Can you work these out from the model? Positions are in its coordinate system, mm. Face numbers are marked on the shaded views. A direction names the side the tool comes from. Give positions to 0.01 mm unless a question says otherwise; leave off trailing zeros. Return JSON: item names as keys, results as strings.
```python
from build123d import *

# Parameters (mm, degrees)
OUTER_R                               = 19.05
BODY_DEPTH                            = 4.7625
F_4_40_TAPPED_HOLE_D                  = 2.2606
SCREW_HOLES_COUNT                     = 4
F_43_0_089_DIAMETER_HOLE1_D           = 2.2606
F_1_8_0_125_DIAMETER_HOLE1_AT_2_COUNT = 2
F_1_8_0_125_DIAMETER_HOLE1_AT_2_PITCH = 19.763158772
F_1_8_0_125_DIAMETER_HOLE2_AT_2_COUNT = 2
F_1_8_0_125_DIAMETER_HOLE2_AT_2_PITCH = 19.763158772
IO_HOLES_PATTERN_COUNT                = 4
INSET_R                               = 19.05
INSET_R_2                             = 11.938
INSET_CUT_DEPTH                       = 1.016
POST_BOTTOMS_COUNT                    = 4
FLAT_CUT_SKETCH_W                     = 2.54
FLAT_CUT_SKETCH_H                     = 38.1
FLAT_CUT_DEPTH                        = 28.358479604


# Read off the part's stored shape, not the designer's step: #36 (0.1065) Diameter Hole1
with BuildPart() as part:
    # outer → Body (new body)
    with BuildSketch(Plane(origin=(0, 0, 0), x_dir=(1, 0, 0), z_dir=(0, 1, 0))):
        with Locations(Location((0, 0, 0), (0, 0, 270))):
            Circle(OUTER_R)
    extrude(amount=-BODY_DEPTH)

    # #4-40 Tapped Hole (through all)
    with Locations(Plane(origin=(0, 0, 0), x_dir=(1, 0, 0), z_dir=(0, 1, 0))):
        with Locations((-11.85393808, 11.85393808)):
            f_4_40_tapped_hole = Hole(F_4_40_TAPPED_HOLE_D / 2)

    # Screw Holes: #4-40 Tapped Hole ×4 about axis
    screw_holes_axis = Axis((0, 0, 0), (0, 1, 0))
    for i in range(1, SCREW_HOLES_COUNT):
        add(f_4_40_tapped_hole.rotate(screw_holes_axis, i * 360 / SCREW_HOLES_COUNT), mode=Mode.SUBTRACT)

    # #43 (0.089) Diameter Hole1 (through all)
    with Locations(Plane(origin=(0, 0, 0), x_dir=(1, 0, 0), z_dir=(0, 1, 0))):
        with Locations((-2.3622, 9.881579386), (-2.3622, -9.881579386)):
            f_43_0_089_diameter_hole1 = Hole(F_43_0_089_DIAMETER_HOLE1_D / 2)

    # Sketch40 → 1/8 (0.125) Diameter Hole1 (revolve, cut)
    with BuildSketch(Plane(origin=(-2.3622, 0, -9.881579386), x_dir=(0, 0, 1), z_dir=(1, 0, 0))):
        Polygon((0, 0), (0, 2.477866233), (1.5875, 1.524), (1.5875, 0), align=None)
    f_1_8_0_125_diameter_hole1 = revolve(axis=Axis((-2.3622, 6.35, -9.881579386), (0, -1, 0)), mode=Mode.SUBTRACT)

    # 1/8 (0.125) Diameter Hole1 at 2: 1/8 (0.125) Diameter Hole1 ×2
    with Locations(*[(0, 0, i * F_1_8_0_125_DIAMETER_HOLE1_AT_2_PITCH) for i in range(1, F_1_8_0_125_DIAMETER_HOLE1_AT_2_COUNT)]):
        add(f_1_8_0_125_diameter_hole1, mode=Mode.SUBTRACT)

    # Sketch42 → 1/8 (0.125) Diameter Hole2 (revolve, cut)
    with BuildSketch(Plane(origin=(-2.3622, -4.7625, -9.881579386), x_dir=(0, 0, -1), z_dir=(1, 0, 0))):
        Polygon((0, 0), (0, 2.477866233), (1.5875, 1.524), (1.5875, 0), align=None)
    f_1_8_0_125_diameter_hole2 = revolve(axis=Axis((-2.3622, -11.1125, -9.881579386), (0, 1, 0)), mode=Mode.SUBTRACT)

    # 1/8 (0.125) Diameter Hole2 at 2: 1/8 (0.125) Diameter Hole2 ×2
    with Locations(*[(0, 0, i * F_1_8_0_125_DIAMETER_HOLE2_AT_2_PITCH) for i in range(1, F_1_8_0_125_DIAMETER_HOLE2_AT_2_COUNT)]):
        add(f_1_8_0_125_diameter_hole2, mode=Mode.SUBTRACT)

    # IO Holes Pattern: #43 (0.089) Diameter Hole1, 1/8 (0.125) Diameter Hole1, 1/8 (0.125) Diameter Hole2 ×4 about axis
    io_holes_pattern_axis = Axis((0, 0, 0), (0, 1, 0))
    add([f_43_0_089_diameter_hole1.rotate(io_holes_pattern_axis, i * 360 / IO_HOLES_PATTERN_COUNT) for i in range(1, IO_HOLES_PATTERN_COUNT)], mode=Mode.SUBTRACT)
    add([f_1_8_0_125_diameter_hole1.rotate(io_holes_pattern_axis, i * 360 / IO_HOLES_PATTERN_COUNT) for i in range(1, IO_HOLES_PATTERN_COUNT)], mode=Mode.SUBTRACT)
    add([f_1_8_0_125_diameter_hole2.rotate(io_holes_pattern_axis, i * 360 / IO_HOLES_PATTERN_COUNT) for i in range(1, IO_HOLES_PATTERN_COUNT)], mode=Mode.SUBTRACT)

    # IO Holes Pattern copy 1 sketch → IO Holes Pattern copy 1 (revolve, cut)
    with BuildSketch(Plane(origin=(9.881579386, 0, 2.3622), x_dir=(1, 0, 0), z_dir=(0, 0, -1))):
        Polygon((0, 0), (0, 2.477866233), (1.5875, 1.524), (1.5875, 0), align=None)
    revolve(axis=Axis((9.881579386, 6.35, 2.3622), (0, -1, 0)), mode=Mode.SUBTRACT)

    # IO Holes Pattern copy 2 sketch → IO Holes Pattern copy 2 (revolve, cut)
    with BuildSketch(Plane(origin=(2.3622, 0, -9.881579386), x_dir=(0, 0, -1), z_dir=(-1, 0, 0))):
        Polygon((0, 0), (0, 2.477866233), (1.5875, 1.524), (1.5875, 0), align=None)
    revolve(axis=Axis((2.3622, 6.35, -9.881579386), (0, -1, 0)), mode=Mode.SUBTRACT)

    # IO Holes Pattern copy 3 sketch → IO Holes Pattern copy 3 (revolve, cut)
    with BuildSketch(Plane(origin=(-9.881579386, 0, -2.3622), x_dir=(-1, 0, 0), z_dir=(0, 0, 1))):
        Polygon((0, 0), (0, 2.477866233), (1.5875, 1.524), (1.5875, 0), align=None)
    revolve(axis=Axis((-9.881579386, 6.35, -2.3622), (0, -1, 0)), mode=Mode.SUBTRACT)

    # IO Holes Pattern copy 4 sketch → IO Holes Pattern copy 4 (revolve, cut)
    with BuildSketch(Plane(origin=(9.881579386, -4.7625, 2.3622), x_dir=(-1, 0, 0), z_dir=(0, 0, -1))):
        Polygon((0, 0), (0, 2.477866233), (1.5875, 1.524), (1.5875, 0), align=None)
    revolve(axis=Axis((9.881579386, -11.1125, 2.3622), (0, 1, 0)), mode=Mode.SUBTRACT)

    # IO Holes Pattern copy 5 sketch → IO Holes Pattern copy 5 (revolve, cut)
    with BuildSketch(Plane(origin=(2.3622, -4.7625, -9.881579386), x_dir=(0, 0, 1), z_dir=(-1, 0, 0))):
        Polygon((0, 0), (0, 2.477866233), (1.5875, 1.524), (1.5875, 0), align=None)
    revolve(axis=Axis((2.3622, -11.1125, -9.881579386), (0, 1, 0)), mode=Mode.SUBTRACT)

    # IO Holes Pattern copy 6 sketch → IO Holes Pattern copy 6 (revolve, cut)
    with BuildSketch(Plane(origin=(-9.881579386, -4.7625, -2.3622), x_dir=(1, 0, 0), z_dir=(0, 0, 1))):
        Polygon((0, 0), (0, 2.477866233), (1.5875, 1.524), (1.5875, 0), align=None)
    revolve(axis=Axis((-9.881579386, -11.1125, -2.3622), (0, 1, 0)), mode=Mode.SUBTRACT)

    # Inset → Inset Cut (cut)
    with BuildSketch(Plane(origin=(0, 0, 0), x_dir=(1, 0, 0), z_dir=(0, 1, 0))):
        with Locations(Location((0, 0, 0), (0, 0, 270))):
            Circle(INSET_R)
        with Locations(Location((0, 0, 0), (0, 0, 270))):
            Circle(INSET_R_2, mode=Mode.SUBTRACT)
    extrude(amount=-INSET_CUT_DEPTH, mode=Mode.SUBTRACT)

    # #36 (0.1065) Diameter Hole1 outline → #36 (0.1065) Diameter Hole1 (revolve, cut)
    with BuildSketch(Plane(origin=(-5.334, 0, -5.334), x_dir=(1, 0, 0), z_dir=(0, 0, 1))):
        Polygon((0, 0), (0, -1.82869403), (1.35255, -1.016), (1.35255, 0), align=None)
    f_36_0_1065_diameter_hole1 = revolve(axis=Axis((-5.334, 0, -5.334), (0, 1, 0)), mode=Mode.SUBTRACT)

    # 36 _0.1065_ Diameter Hole1 2 outline → 36 _0.1065_ Diameter Hole1 2 (revolve, cut)
    with BuildSketch(Plane.XY.offset(-5.334)):
        Polygon((0, 0), (0, -1.82869403), (1.35255, -1.016), (1.35255, 0), align=None)
    f_36_0_1065_diameter_hole1_2 = revolve(axis=Axis((0, 0, -5.334), (0, 1, 0)), mode=Mode.SUBTRACT)

    # Post Bottoms: #36 (0.1065) Diameter Hole1, 36 _0.1065_ Diameter Hole1 2 ×4 about axis
    post_bottoms_axis = Axis((0, 0, 0), (0, 1, 0))
    add([f_36_0_1065_diameter_hole1.rotate(post_bottoms_axis, i * 360 / POST_BOTTOMS_COUNT) for i in range(1, POST_BOTTOMS_COUNT)], mode=Mode.SUBTRACT)
    add([f_36_0_1065_diameter_hole1_2.rotate(post_bottoms_axis, i * 360 / POST_BOTTOMS_COUNT) for i in range(1, POST_BOTTOMS_COUNT)], mode=Mode.SUBTRACT)

    # v_sketch → V cut (revolve, cut)
    with BuildSketch(Plane.XY, mode=Mode.PRIVATE) as v_cut_sk:
        Polygon((-13.97, -1.397), (-13.335909517, -1.016), (-14.604090483, -1.016), align=None)
    revolve(v_cut_sk.sketch.rotate(Axis((0, 0.15875, 0), (0, -1, 0)), 270), axis=Axis((0, 0.15875, 0), (0, -1, 0)), mode=Mode.SUBTRACT)

    # Flat Cut Sketch → Flat Cut (cut, through all)
    with BuildSketch(Plane(origin=(0, 0, 0), x_dir=(1, 0, 0), z_dir=(0, 1, 0))):
        with Locations((19.05, 0)):
            Rectangle(FLAT_CUT_SKETCH_W, FLAT_CUT_SKETCH_H)
        with Locations((-19.05, 0)):
            Rectangle(FLAT_CUT_SKETCH_W, FLAT_CUT_SKETCH_H)
    extrude(amount=-FLAT_CUT_DEPTH, mode=Mode.SUBTRACT)


solid = part.part
```
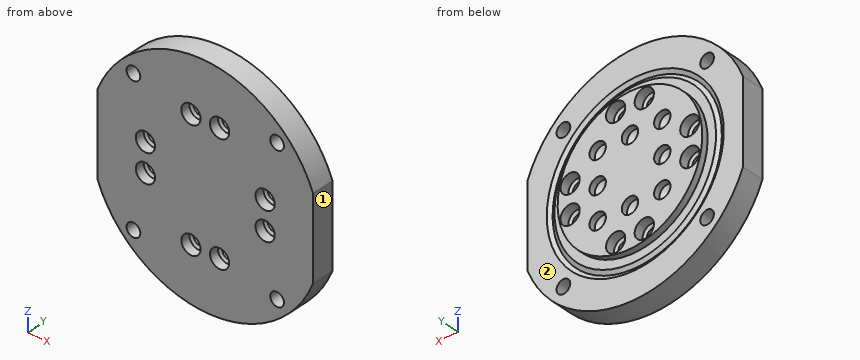
1. On a 3-axis mill with a long thin cutter (end or side, diameter ignored), from which of +Z, -Z, +X, -X, +Y, -Y can I reach the whole of each face in a straight line? I mean the marked faces 1 and 2. Say none if no direction works.
Checks:
{"face 1": "+Z, -Z, +X, +Y, -Y", "face 2": "+Y"}
2. Suppose I cut it at A-A (y = -3.9). State how many separate pieces and enclosed holes the cut face has, plus the area to 3 significant figures.
Checks:
{"separate pieces": "1", "enclosed holes": "12", "area": "1,040 mm^2"}
3. For pin 1 Ø2 at (x, y) = (-6.5, -0.5) entering from -Z; pin 2 Ø3 at (x, z) = (9.88, -2.36) entering from -Y; pin 3 Ø2.5 at (x, z) = (-9.88, -2.36) entering from -Y; pin 4 Ø2 at (x, z) = (11.85, -11.85) entering from +Y, each with a flat end and sliding along its axis, tell me the tip position at first contact or that it passes through.
Checks:
{"pin 1": "z = -18.19", "pin 2": "y = -3.19", "pin 3": "y = -3.04", "pin 4": "through"}
4. If I drill on L1, parallel to X at y = -0.3, z = 6; L2, parallel to Z at x = 10.5, y = -2.4; L3, parallel to Z at x = -5, y = -0.5, over which ranges is the centre line in solid material (lowest first)? Write a range as [from, to].
Checks:
{"L1": "[-10.32, -6.51], [-4.16, -1.18], [1.18, 4.16], [6.51, 10.32]", "L2": "[-15.9, -3.31], [-1.42, 1.42], [3.31, 15.9]", "L3": "[-10.84, -6.64], [-4.02, -1.31], [1.31, 4.02], [6.64, 10.84]"}
